For this review, use the dimensioned drawing (mm, ordinates from the lowest corner) and the shaded views. Coordinates: 2 decimals unless noted, no trailing zeros. Write each loop counter-clockwise with the first axis right and the second up, starting at its lowest first coordinate (ties: lowest second). Pieces come first, ordered by that corner, then holes. Notation, with made-up numbers: M 47.5,-17.75 L 89.5,-17.75 A17 cw 89.5,0.25 Z; hole C 85,24.25 d8. An arc over 180 degrees is marked long. One line per question, with ' | ' between items.
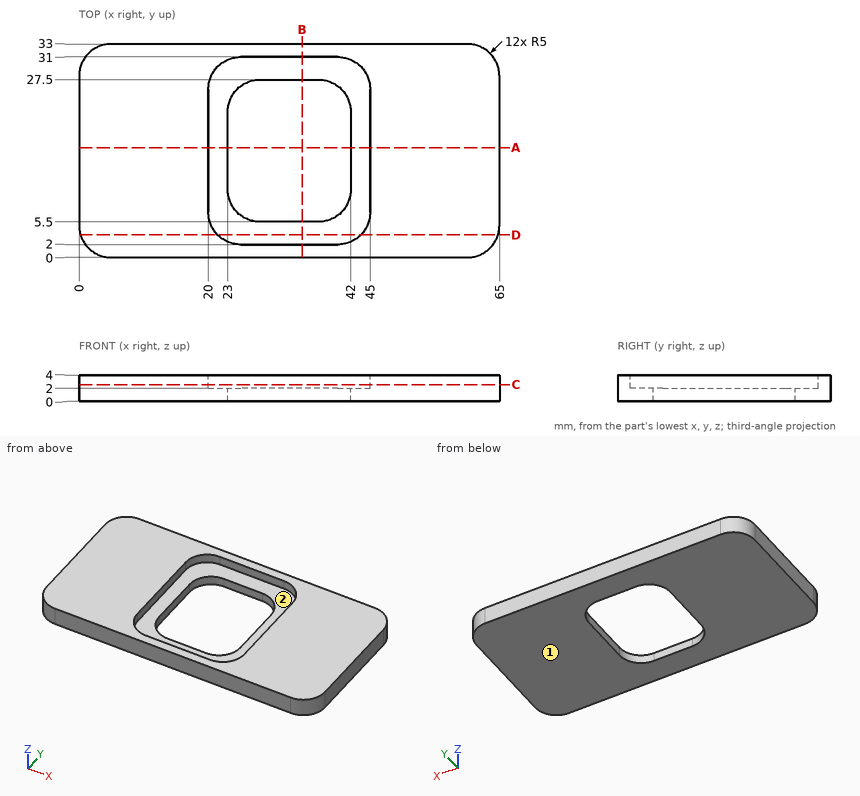
1. Draft analysis for pull direction Y (two halves, no side actions). For the marked faces 1 and 2, state which applies: pulls with the +Y half, pulls with the -Y half, needs draft (parallel to the pull), parting line crosses it, or undercut.
Answer sheet:
face 1: needs draft | face 2: undercut
2. To check wall thickness, follow line 1 along X through (y, z) = (7.5, 2.45); line 2 along Y through (x, z) = (29, 0.65); line 3 along X through (y, z) = (15.5, 0.4). State the ranges of each line that lie inside material, in increasing order. Write a range as [from, to].
Answer sheet:
line 1: [0, 20], [45, 65] | line 2: [0, 5.5], [27.5, 33] | line 3: [0, 23], [42, 65]
3. Take a section at D-D (y = 3.5). Write out the cut boundary in (x, z).
Answer sheet:
outline: M 0.23,0 L 64.77,0 L 64.77,4 L 43.57,4 L 43.57,2 L 21.43,2 L 21.43,4 L 0.23,4 Z
4. Take a section at A-A (y = 17). Write out the cut boundary in (x, z).
Answer sheet:
outline: M 0,0 L 23,0 L 23,2 L 20,2 L 20,4 L 0,4 Z; M 42,0 L 65,0 L 65,4 L 45,4 L 45,2 L 42,2 Z
5. Take a section at B-B (x = 34.5). Write out the cut boundary in (y, z).
Answer sheet:
outline: M 0,0 L 5.5,0 L 5.5,2 L 2,2 L 2,4 L 0,4 Z; M 27.5,0 L 33,0 L 33,4 L 31,4 L 31,2 L 27.5,2 Z
6. Take a section at C-C (z = 2.6). Write out the cut boundary in (x, y), then the cut area to 3 significant figures.
Answer sheet:
outline: M 0,5 A5 ccw 5,0 L 60,0 A5 ccw 65,5 L 65,28 A5 ccw 60,33 L 5,33 A5 ccw 0,28 Z; hole M 20,7 A5 ccw 25,2 L 40,2 A5 ccw 45,7 L 45,26 A5 ccw 40,31 L 25,31 A5 ccw 20,26 Z | area: 1,420 mm^2
7. Insertion check: pin 1 Ø12.5 at (x, y) = (29, 9.5) entering from +Z; pin 2 Ø3 at (x, y) = (58, 15) entering from -Z. Each pin has a flat end and moves straight along its axis. Give the tip position at first contact, or say it passes through.
Answer sheet:
pin 1: z = 2 | pin 2: z = 0
